```python
from build123d import *

# Parameters (mm, degrees)
F0_R     = 1.87325
F1_DEPTH = 5.999988
F2_R     = 5.99948
F3_DEPTH = 5.999988
F4_R     = 1.27
F5_DEPTH = 12.000976


with BuildPart() as f1:
    # F0 (on Top) → F1 (new body)
    with BuildSketch(Plane.XY):
        with Locations((-128.226578, -56.971956)):
            Circle(F0_R)
    extrude(amount=F1_DEPTH)

    # F2 (on face) → F3 (join)
    with BuildSketch(Plane.XY.offset(5.999988)):
        with Locations((-128.226578, -56.971956)):
            Circle(F2_R)
    extrude(amount=F3_DEPTH)

    # F4 (on face) → F5 (cut, through all)
    with BuildSketch(Plane.XY.offset(11.999976)):
        with Locations((-128.226578, -56.971956)):
            Circle(F4_R)
    extrude(amount=-F5_DEPTH, mode=Mode.SUBTRACT)


solid = f1.part
```
Read the model definition and answer for the solid it produces. Units are mm, in the model's axes. A direction names the side the tool comes from. Round coordinates to 2 decimals unless told otherwise and drop trailing zeros. Loops run counter-clockwise (first coordinate to the right, second up) from the corner with the lowest first, then second, coordinate; pieces in that order, holes last. Notation, with made-up numbers: (55, 86.25) -> (112, 86.25) arc R16 ccw to (112, 116.25) -> close; hole circle Ø10 at (-2.75, 9). An arc over 180 degrees is marked (long way). One line per item, written item: value.
1) A cutting plane is placed at A-A (x = -127.75). Determine the outline of the cut face in (y, z).
Answer list:
outline: (-62.95, 6) -> (-58.78, 6) -> (-58.78, 0) -> (-58.15, 0) -> (-58.15, 12) -> (-62.95, 12) -> close; (-55.79, 0) -> (-55.16, 0) -> (-55.16, 6) -> (-50.99, 6) -> (-50.99, 12) -> (-55.79, 12) -> close
2) For faces 4 (the face through (-130.1, -56.9, 3)), 5 (the face through (-128.31, -55.55, 12)), determine the directions among +Z, -Z, +X, -X, +Y, -Y from which every point of the face is accessible in a straight line to the end or side of a thin tool.
Answer list:
face 4: -Z
face 5: +Z, +X, -X, +Y, -Y
3) A cutting plane is placed at D-D (x = -125.5). Determine the outline of the cut face in (y, z), and give its area (3 significant figures).
Answer list:
outline: (-62.32, 6) -> (-51.63, 6) -> (-51.63, 12) -> (-62.32, 12) -> close
area: 64.1 mm²
4) A cutting plane is placed at C-C (y = -53.5). Determine the outline of the cut face in (x, z), and give its area (3 significant figures).
Answer list:
outline: (-133.12, 6) -> (-123.33, 6) -> (-123.33, 12) -> (-133.12, 12) -> close
area: 58.7 mm²
5) Flat-ended cylindrical pins translate along their axes: P1, Ø4, axis at x = -124, z = 4.5, coming from the +Y side; P2, Ø4, axis at x = -131, z = 4.5, coming from the -Y side; P3, Ø3, axis at y = -54.5, z = 5, coming from the +X side; P4, Ø4, axis at y = -61, z = 2, coming from the +X side. Find the tip coordinate at first contact, or state that the pin passes through.
Answer list:
P1: stops at y = -51.72
P2: stops at y = -62.79
P3: stops at x = -122.38
P4: passes through
6) A cutting plane is placed at B-B (z = 4.75). Determine the outline of the cut face in (x, y).
Answer list:
outline: circle Ø3.75 at (-128.23, -56.97); hole circle Ø2.54 at (-128.23, -56.97)
7) The mould has two halves that part along X. Classify faces 1 (the face through (-129.234, -57.745, 6.084)), 2 (the face through (-130, -58, 6)), 3 (the face through (-129.53, -62.83, 8.96)): pulls with the +X half, pulls with the -X half, needs draft (parallel to the pull), parting line crosses it, or undercut.
Answer list:
face 1: undercut
face 2: needs draft
face 3: parting line crosses it
8) Consider L1, parallel to Z at x = -126, y = -58.75; L2, parallel to X at y = -58, z = 11.5; L3, parallel to X at y = -57.25, z = 7.25. Determine where each line is inside the solid, lowest interval first. Write a range as [from, to].
Answer list:
L1: z = [6, 12]
L2: x = [-134.14, -128.97], [-127.48, -122.32]
L3: x = [-134.22, -129.47], [-126.99, -122.23]
